Design review of the part built by this model. Coordinates are the model's own, in mm. Face numbers are marked on the shaded views. A direction names the side the tool comes from. Coordinates: 2 decimals unless noted, no trailing zeros. Loops run counter-clockwise (first coordinate to the right, second up) from the corner with the lowest first, then second, coordinate; pieces in that order, holes last. Notation, with made-up numbers: (29, 43) - (39, 43) arc R31 ccw to (39, 79) - close; hole circle Ø3 at (10, 44). An arc over 180 degrees is marked (long way). One line per question, with ' | ' between items.
Autodesk Inventor part; units mm, degrees
ref_plane "YZ Plane" through (0, 0, 0) normal (1, 0, 0) x (0, 1, 0)
ref_plane "XZ Plane" through (0, 0, 0) normal (0, 1, 0) x (-1, 0, 0)
ref_plane "XY Plane" through (0, 0, 0) normal (0, 0, 1) x (1, 0, 0)
sketch "Sketch1" plane through (0, 0, 0) normal (0, 0, 1) x (1, 0, 0)
  line L0 (-36.4, 0) -> (36.4, 0) construction
  line L1 (0, -36.4) -> (0, 36.4) construction
  circle A0 centre (0, 0) radius 26
  dimension "d0" = 52
extrude "Выдавливание1" add sketch "Sketch1" along normal blind 10
hole "Отверстие1" at (0, 0, 10) direction (0, 0, -1) diameter 31.3762 end through all
sketch "Sketch2" plane through (0, 0, 10) normal (0, 0, 1) x (1, 0, 0)
  circle A0 centre (0, 0) radius 26
  circle A1 centre (0, 0) radius 21 construction
  line L0 (-36.4, 0) -> (36.4, 0) construction
  line L1 (0, -36.4) -> (0, 36.4) construction
  point P0 (-21, 0)
  point P1 (0, 21)
  point P2 (21, 0)
  point P3 (0, -21)
  dimension "d13" = 42
hole "Отверстие2" at (-21, 0, 10) at (0, 21, 10) at (21, 0, 10) at (0, -21, 10) direction (0, 0, -1) diameter 4.5 depth 7 tip angle 118
chamfer "Фаска1" distance 0.6 angle 45 4 edges at (0, -18.75, 10) (-21, 2.25, 10) (21, 2.25, 10) (0, 23.25, 10)
chamfer "Фаска2" distance 1 angle 45 2 edges at (-26, 0, 10) (-26, 0, 0)
sketch "Sketch3" plane through (0, 0, 0) normal (1, 0, 0) x (0, 1, 0)
  line L0 (-15.6881, 0) -> (-15.6881, 10) construction
  line L1 (15.6881, 0) -> (15.6881, 10) construction
  line L2 (-16.5, 10) -> (0, -6.5)
  line L3 (-16.5, 10) -> (0, 10)
  line L4 (0, 10) -> (0, -6.5)
  line L5 (0, -11.1) -> (0, 21.1) construction
  line L6 (-15.6074, 5) -> (15.0846, 5) construction
  line L7 (-22.9376, 0) -> (22.1257, 0) construction
  line L8 (-16.5, 0) -> (0, 16.5)
  line L9 (-16.5, 0) -> (0, 0)
  line L10 (0, 0) -> (0, 16.5)
  point P0 (15.6881, 5)
  dimension "d30" = 10
  dimension "d31" = 33
  dimension "d32" = 45
  dimension "d34" = 5
revolve "Вращение1" cut sketch "Sketch3" angle 360 about axis through (0, 0, -10) along (0, 0, 1)
equation "\"d0\" = D_L"
equation "\"d2\" = m_"
equation "\"d13\" = D_x"
equation "\"d14\" = d1"
equation "\"d16\" = d1"
equation "\"d19\" = h_"
equation "\"d21\" = c1"
equation "\"d24\" = c_"
equation "\"d30\" = m_"
equation "\"d31\" = d_"
equation "\"d34\" = 0.5 * m_"
equation "\"d_\" = 33"
equation "\"D_L\" = 52"
equation "\"D_x\" = 42"
equation "\"d1\" = 4.5"
equation "\"m_\" = 10"
equation "\"h_\" = 7"
equation "\"c_\" = 1"
equation "\"c1\" = 0.6"
properties part number "Гайка M33x1.5 6H ГОСТ 6393-73" material "Сталь, мягкая"
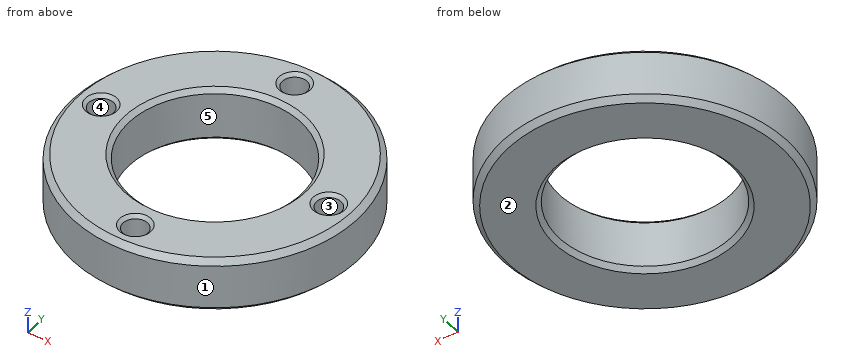
Q1. Tool access review of the marked faces 4 and 5: name each direction out of +Z, -Z, +X, -X, +Y, -Y from which nothing blocks a thin tool from reaching the whole face with its end or side.
Returned:
face 4: +Z | face 5: +Z, -Z
Q2. Take a section at A-A (z = 5.5). Give the boundary of the cut face in (x, y).
Returned:
outline: circle Ø52 at (0, 0); hole circle Ø4.5 at (-21, 0); hole circle Ø31.38 at (0, 0); hole circle Ø4.5 at (0, -21); hole circle Ø4.5 at (0, 21); hole circle Ø4.5 at (21, 0)
Q3. To check wall thickness, follow line 1 along Y through (x, z) = (1, 3.25); line 2 along Y through (x, z) = (2, 4.5); line 3 along Y through (x, z) = (-21, 4.5). State the ranges of each line that lie inside material, in increasing order.
Returned:
line 1: y = -25.98 to -23.02, -18.98 to -15.66, 15.66 to 18.98, 23.02 to 25.98 | line 2: y = -25.92 to -22.03, -19.97 to -15.56, 15.56 to 19.97, 22.03 to 25.92 | line 3: y = -15.33 to -2.25, 2.25 to 15.33
Q4. For pin 1 (1.5 mm diameter, centred on y = 9.5, z = 7, fed in from +X); pin 2 (1.5 mm diameter, centred on x = -14.5, z = 8, fed in from -Y); pin 3 (3 mm diameter, centred on x = 3.5, z = 4.5, fed in from +Y), all flat-tipped, find the tip position at first contact; note any pin that passes through.
Returned:
pin 1: stops at x = 24.48 | pin 2: stops at y = -22.07 | pin 3: stops at y = 25.92
Q5. Draft analysis for pull direction Y (two halves, no side actions). For the marked faces 1, 2 and 3, state which applies: +Y half, -Y half, draft (parallel to the pull), parting line (faces both ways), or undercut.
Returned:
face 1: parting line | face 2: draft | face 3: undercut
